Here's how the part is built. I have some questions about the finished solid (model axes, mm). Face numbers are marked on the shaded views. A direction names the side the tool comes from. Round coordinates to 2 decimals unless told otherwise and drop trailing zeros. Loops run counter-clockwise (first coordinate to the right, second up) from the corner with the lowest first, then second, coordinate; pieces in that order, holes last. Notation, with made-up numbers: M 42.25,11.5 L 88.25,11.5 A21 ccw 88.25,30.5 Z; hole C 32,6 d1. An arc over 180 degrees is marked long. Answer as CSV lines item,"result".
```python
from build123d import *

# Parameters (mm, degrees)
SKETCH1_W            = 70
SKETCH1_H            = 50
BOSS_EXTRUDE1_DEPTH  = 6.35
SKETCH2_W            = 60
SKETCH2_H            = 40
CUT_EXTRUDE1_DEPTH   = 3.175
DIVIDERS_DEPTH       = 2.5
SKETCH11_W           = 0.5
SKETCH11_H           = 0.5
SKETCH11_W_2         = 4.089905709
SKETCH11_W_3         = 3.608523714
SKETCH11_H_2         = 3.849214712
BOSS_EXTRUDE3_DEPTH  = 0.1
LPATTERN1_COUNT      = 3
LPATTERN1_PITCH      = 20
LPATTERN1_COUNT_DIR2 = 2
LPATTERN1_PITCH_DIR2 = 20
FILLET1_R            = 2


with BuildPart() as part:
    # Sketch1 → Boss-Extrude1 (new body)
    with BuildSketch(Plane(origin=(0, 0, 0), x_dir=(1, 0, 0), z_dir=(0, 1, 0))):
        Rectangle(SKETCH1_W, SKETCH1_H)
    extrude(amount=BOSS_EXTRUDE1_DEPTH)

    # Sketch2 → Cut-Extrude1 (cut)
    with BuildSketch(Plane(origin=(0, 6.35, 0), x_dir=(1, 0, 0), z_dir=(0, 1, 0))):
        Rectangle(SKETCH2_W, SKETCH2_H)
    extrude(amount=-CUT_EXTRUDE1_DEPTH, mode=Mode.SUBTRACT)

    # Sketch10 → Dividers (add)
    with BuildSketch(Plane(origin=(0, 3.175, 0), x_dir=(1, 0, 0), z_dir=(0, 1, 0))):
        Polygon((-10.25, -0.25), (-10.25, -20), (-9.75, -20), (-9.75, -0.25), (9.818560524, -0.25), (9.681439476, -20), (10.181439476, -20), (10.318560524, -0.25), (30, -0.25), (30, 0.25), (10.318560524, 0.25), (10.318560524, 20), (9.818560524, 20), (9.818560524, 0.25), (-9.75, 0.25), (-9.75, 20), (-10.25, 20), (-10.25, 0.25), (-30, 0.25), (-30, -0.25), align=None)
    extrude(amount=DIVIDERS_DEPTH)

    # Sketch11 → Boss-Extrude3 (add)
    with BuildSketch(Plane(origin=(0, 3.175, 0), x_dir=(1, 0, 0), z_dir=(0, 1, 0))):
        with Locations((-20.125, 10.125)):
            Rectangle(SKETCH11_W, SKETCH11_H)
        with Locations((-22.419952854, 10.125)):
            Rectangle(SKETCH11_W_2, SKETCH11_H)
        with Locations((-18.070738143, 10.125)):
            Rectangle(SKETCH11_W_3, SKETCH11_H)
        with BuildLine():
            ThreePointArc((-24.464905709, 10.375), (-26.024839917, 10.125), (-24.464905709, 9.875))
            Line((-24.464905709, 9.875), (-24.464905709, 10.375))
        make_face()
        with Locations((-20.125, 12.299607356)):
            Rectangle(SKETCH11_W, SKETCH11_H_2)
        with BuildLine():
            Line((-16.266476286, 10.375), (-16.266476286, 9.875))
            ThreePointArc((-16.266476286, 9.875), (-14.706542078, 10.125), (-16.266476286, 10.375))
        make_face()
        with BuildLine():
            ThreePointArc((-19.875, 14.224214712), (-20.125, 15.784148919), (-20.375, 14.224214712))
            Line((-20.375, 14.224214712), (-19.875, 14.224214712))
        make_face()
    boss_extrude3 = extrude(amount=BOSS_EXTRUDE3_DEPTH)

    # LPattern1: Boss-Extrude3 3 × 2
    with Locations(*[(i * LPATTERN1_PITCH, 0, j * LPATTERN1_PITCH_DIR2) for i in range(LPATTERN1_COUNT) for j in range(LPATTERN1_COUNT_DIR2) if (i, j) != (0, 0)]):
        add(boss_extrude3)

    # Fillet1
    fillet1_edges = [part.edges().sort_by_distance(p)[0] for p in [
        (35, 3.175, 25),
        (-35, 3.175, 25),
        (-35, 3.175, -25),
        (35, 3.175, -25),
    ]]
    fillet(fillet1_edges, radius=FILLET1_R)


solid = part.part
```
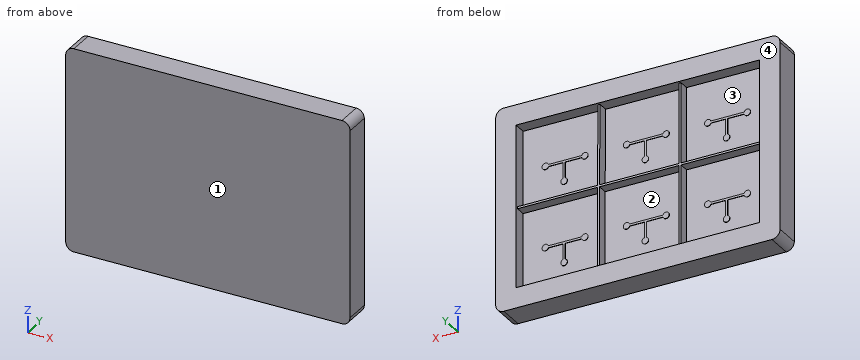
1. We'd pull the mould along Z, two halves only. Please class the marked faces 1 and 2: pulls with the +Z half, pulls with the -Z half, needs draft (parallel to the pull), parting line crosses it, or undercut.
Evaluation:
face 1,"needs draft"
face 2,"undercut"
2. If I drill on line 1 (X direction, y = 4.25, z = -4); line 2 (Z direction, x = 28, y = 4.75); line 3 (Z direction, x = -22, y = 5.75), over which ranges is the centre line in solid material (lowest first)? Write a range as [from, to].
Evaluation:
line 1,"x = [-35, -30], [-10.25, -9.75], [9.82, 10.32], [30, 35]"
line 2,"z = [-25, -20], [-0.25, 0.25], [20, 25]"
line 3,"z = [-25, -20], [20, 25]"
3. For P1, Ø5, axis at x = -21, z = -13.5, coming from the +Y side (3 decimals); P2, Ø16, axis at x = 17.5, z = 7, coming from the +Y side (3 decimals), each with a flat end and sliding along its axis, tell me the tip position at first contact or that it passes through.
Evaluation:
P1,"stops at y = 3.275"
P2,"stops at y = 5.675"
4. I want a section at C-C, the plane x = 6. Please give me the cut outline in (y, z) (3 decimals), and give its area (3 significant figures).
Evaluation:
outline,"M 0,-25 L 6.35,-25 L 6.35,-20 L 3.175,-20 L 3.175,-0.25 L 5.675,-0.25 L 5.675,0.25 L 3.175,0.25 L 3.175,20 L 6.35,20 L 6.35,25 L 0,25 Z"
area,"192 mm²"
5. I want a section at D-D, the plane z = -12. Please give me the cut outline in (x, y) (3 decimals).
Evaluation:
outline,"M -35,0 L 35,0 L 35,6.35 L 30,6.35 L 30,3.175 L 20.125,3.175 L 20.125,3.275 L 19.625,3.275 L 19.625,3.175 L 10.319,3.175 L 10.319,5.675 L 9.819,5.675 L 9.819,3.175 L 0.125,3.175 L 0.125,3.275 L -0.375,3.275 L -0.375,3.175 L -9.75,3.175 L -9.75,5.675 L -10.25,5.675 L -10.25,3.175 L -19.875,3.175 L -19.875,3.275 L -20.375,3.275 L -20.375,3.175 L -30,3.175 L -30,6.35 L -35,6.35 Z"
6. Which directions (+Z, -Z, +X, -X, +Y, -Y) give clear straight access to the entire face, cutting with the end or side of a thin tool? Please do the marked faces 3 and 4.
Evaluation:
face 3,"+Y"
face 4,"+Z, -Z, +X, -X, +Y"
7. I want a section at B-B, the plane z = -5.5. Please give me the cut outline in (x, y) (3 decimals).
Evaluation:
outline,"M -35,0 L 35,0 L 35,6.35 L 30,6.35 L 30,3.175 L 10.319,3.175 L 10.319,5.675 L 9.819,5.675 L 9.819,3.175 L -9.75,3.175 L -9.75,5.675 L -10.25,5.675 L -10.25,3.175 L -30,3.175 L -30,6.35 L -35,6.35 Z"
8. I want a section at A-A, the plane y = 4.25. Count the separate pieces of the cut face and the enclosed holes in it, and give its area (3 significant figures).
Evaluation:
separate pieces,"1"
enclosed holes,"6"
area,"1,170 mm²"
